Source: CAD feature listing. Evaluate the final solid. Frame: model axes, mm. Face numbers are marked on the shaded views. A direction names the side the tool comes from. Give positions to 0.01 mm unless a question says otherwise; leave off trailing zeros. Loops run counter-clockwise (first coordinate to the right, second up) from the corner with the lowest first, then second, coordinate; pieces in that order, holes last. Notation, with made-up numbers: M 17,1 L 25,1 A14 cw 25,26 Z; hole C 46.25,53.25 d11. An arc over 180 degrees is marked long. Write item = value, one per line.
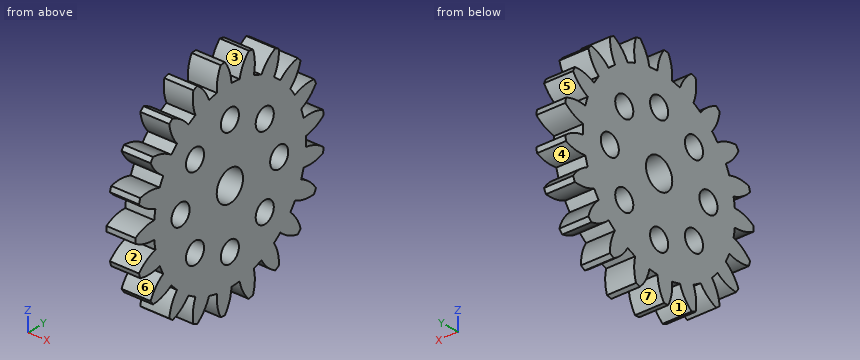
from build123d import *

# Parameters (mm, degrees)
BASPROSKE_W         = 3
BASPROSKE_H         = 11.5
TOOTHCUT_DEPTH      = 17.537835409
TEETHCUTS_COUNT     = 21
TEETHCUTS_ANGLE     = 342.857142857
BORSKE_R            = 4
BORE_DEPTH          = 50.0000508
EXTRUDE_START       = -3
SKETCH_1_R          = 4
EXTRUDE_1_DEPTH     = 3
SKETCH_2_R          = 1.6
SKETCH_2_R_2        = 1.1
CUT_EXTRUDE_1_DEPTH = 17.52708436


with BuildPart() as part:
    # BasProSke → Base-Revolve (revolve)
    with BuildSketch(Plane(origin=(0, 0, 0), x_dir=(1, 0, 0), z_dir=(0, 1, 0)), mode=Mode.PRIVATE) as base_revolve_sk:
        with Locations((1.5, 5.75)):
            Rectangle(BASPROSKE_W, BASPROSKE_H)
    revolve(base_revolve_sk.sketch.rotate(Axis((-10, 0, 0), (1, 0, 0)), 180), axis=Axis((-10, 0, 0), (1, 0, 0)))

    # TooCutSke → ToothCut (cut, through all)
    with BuildSketch(Plane(origin=(0, 0, 0), x_dir=(0, 0, -1), z_dir=(1, 0, 0))):
        with BuildLine():
            ThreePointArc((0.49526894, 9.235730057), (0, 9.249), (-0.49526894, 9.235730057))
            ThreePointArc((-0.49526894, 9.235730057), (-0.823521057, 10.404716786), (-1.472455249, 11.430954496))
            ThreePointArc((-1.472455249, 11.430954496), (0, 11.5254), (1.472455249, 11.430954496))
            ThreePointArc((1.472455249, 11.430954496), (0.823521057, 10.404716786), (0.49526894, 9.235730057))
        make_face()
    toothcut = extrude(amount=TOOTHCUT_DEPTH, mode=Mode.SUBTRACT)

    # TeethCuts: ToothCut ×21 about axis
    teethcuts_axis = Axis((-10, 0, 0), (1, 0, 0))
    for i in range(1, TEETHCUTS_COUNT):
        add(toothcut.rotate(teethcuts_axis, i * TEETHCUTS_ANGLE / (TEETHCUTS_COUNT - 1)), mode=Mode.SUBTRACT)

    # BorSke → Bore (cut, symmetric)
    with BuildSketch(Plane(origin=(0, 0, 0), x_dir=(0, 0, -1), z_dir=(1, 0, 0))):
        with Locations(Location((0, 0, 0), (0, 0, 180))):
            Circle(BORSKE_R)
    extrude(amount=BORE_DEPTH, both=True, mode=Mode.SUBTRACT)

    # ｽｹｯﾁ1 → ﾎﾞｽ - 押し出し1 (add)
    with BuildSketch(Plane.ZY.offset(EXTRUDE_START)):
        Circle(SKETCH_1_R)
    extrude(amount=EXTRUDE_1_DEPTH)

    # ｽｹｯﾁ2 → ｶｯﾄ - 押し出し1 (cut, through all)
    with BuildSketch(Plane(origin=(3, 0, 0), x_dir=(0, 0, -1), z_dir=(1, 0, 0))):
        Circle(SKETCH_2_R)
        with Locations((6, 0)):
            Circle(SKETCH_2_R_2)
        with Locations((4.242640687, -4.242640687)):
            Circle(SKETCH_2_R_2)
        with Locations((0, -6)):
            Circle(SKETCH_2_R_2)
        with Locations((-4.242640687, -4.242640687)):
            Circle(SKETCH_2_R_2)
        with Locations((-6, 0)):
            Circle(SKETCH_2_R_2)
        with Locations((-4.242640687, 4.242640687)):
            Circle(SKETCH_2_R_2)
        with Locations((0, 6)):
            Circle(SKETCH_2_R_2)
        with Locations((4.242640687, 4.242640687)):
            Circle(SKETCH_2_R_2)
    extrude(amount=-CUT_EXTRUDE_1_DEPTH, mode=Mode.SUBTRACT)


solid = part.part
1. Reachability of the marked faces 1, 2, 3 and 4 from +Z, -Z, +X, -X, +Y, -Y: full face, straight path, thin tool, end or side. Return the list, or none.
Derived:
face_1 = -Z, +X, -X
face_2 = +X, -X, -Y
face_3 = +Z, +X, -X
face_4 = +X, -X
2. Cut plane A-A, the plane y = 0.5. Return the cut outline in (x, z), then the cut area to 3 significant figures.
Derived:
outline = M 0,-9.24 L 3,-9.24 L 3,-6.98 L 0,-6.98 Z; M 0,-5.02 L 3,-5.02 L 3,-1.52 L 0,-1.52 Z; M 0,1.52 L 3,1.52 L 3,5.02 L 0,5.02 Z; M 0,6.98 L 3,6.98 L 3,9.24 L 0,9.24 Z
area = 34.5 mm²
3. Cut plane C-C, the plane y = 3.5. Return the cut outline in (x, z), then the cut area to 3 significant figures.
Derived:
outline = M 0,-8.56 L 3,-8.56 L 3,-5.05 L 0,-5.05 Z; M 0,-3.43 L 3,-3.43 L 3,3.43 L 0,3.43 Z; M 0,5.05 L 3,5.05 L 3,8.56 L 0,8.56 Z
area = 41.6 mm²
4. Pull-direction query (Y, two-part tool) for the marked faces 5, 6 and 7; classes: +Y half, -Y half, draft (parallel to the pull), parting line (faces both ways), or undercut.
Derived:
face_5 = +Y half
face_6 = -Y half
face_7 = undercut
5. First-contact query: pin 1 Ø1.5 at (x, y) = (1.5, -4) entering from +Z; pin 2 Ø1 at (x, y) = (2.5, 7.5) entering from +Z. Flat tips, straight axial feed; report the tip coordinate or a pass-through.
Derived:
pin_1 = 10.8
pin_2 = 7.96
6. Cut plane B-B, the plane y = 6.5. Return the cut outline in (x, z).
Derived:
outline = M 0,-7.22 L 3,-7.22 L 3,-0.98 L 0,-0.98 Z; M 0,0.98 L 3,0.98 L 3,7.22 L 0,7.22 Z
7. Material intervals for probe 1 along Y at (x, z) = (2, 0); probe 2 along Z at (x, y) = (1.95, 5); probe 3 along Z at (x, y) = (1.75, 0.5), sorted ascending. Write a range as from..to.
Derived:
probe_1 = -11.5..-7.1, -4.9..-1.6, 1.6..4.9, 7.1..9.25
probe_2 = -9.76..-5.04, -3.44..-0.46, 0.46..3.44, 5.04..9.76
probe_3 = -9.24..-6.98, -5.02..-1.52, 1.52..5.02, 6.98..9.24
8. Cut plane D-D, the plane x = 2.6. Count the separate pieces of the cut face and the enclosed holes in it, then the cut area to 3 significant figures.
Derived:
separate_pieces = 1
enclosed_holes = 9
area = 296 mm²
